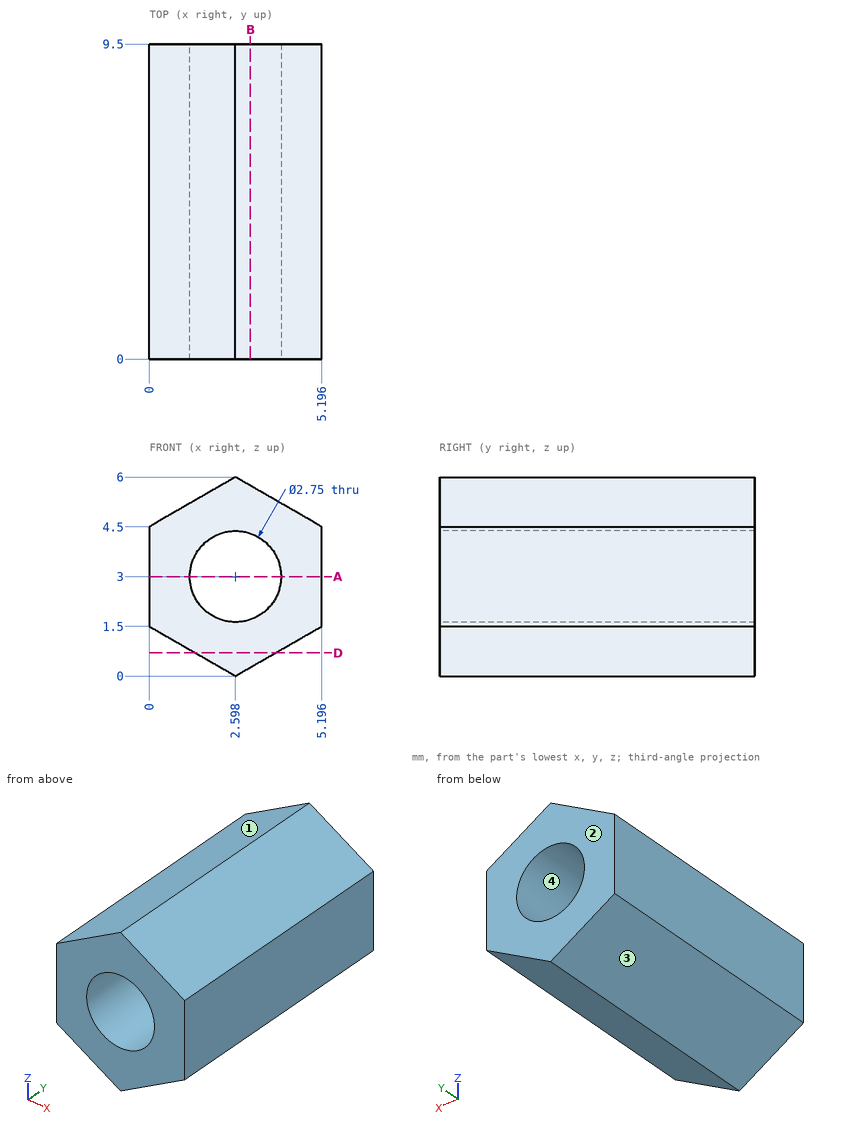
Input: dimensioned drawing with shaded views. Units: mm. Origin: part minimum x, y, z. Round coordinates to 2 decimals unless told otherwise and drop trailing zeros. Order: outer loops, then holes, each group sorted by start corner. A loop starts at its lowest first (then second) coordinate and runs counter-clockwise, first axis right, second up. Notation, with made-up numbers: (2.25, -25.5) -> (29.25, -25.5) arc R34 cw to (29.25, 6.5) -> close; hole circle Ø6 at (63.25, 86). An arc over 180 degrees is marked (long way). Put each result on its own line as item: value. Start each with the question number.
Q1. First-contact query: pin 1 (3 mm diameter, centred on x = 4.5, y = 1.5, fed in from +Z); pin 2 (2 mm diameter, centred on x = 1.5, y = 8, fed in from +Z). Flat tips, straight axial feed; report the tip coordinate or a pass-through.
Q2. Section A-A on z = 3. Return the cut outline in (x, y).
Q3. Section B-B on x = 3.05. Return the cut outline in (y, z).
Q4. Pull-direction query (Z, two-part tool) for the marked faces 1, 2, 3 and 4; classes: +Z half, -Z half, draft (parallel to the pull), parting line (faces both ways), or undercut.
Q5. Line query: probe 1 along Z at (x, y) = (2.2, 2.75); probe 2 along X at (y, z) = (7.5, 2) (1 decimal); probe 3 along Z at (x, y) = (3.4, 7). Output: solid intervals per line, ascending.
Q6. Section D-D on z = 0.7. Return the cut outline in (x, y).
Ans:
1. pin 1: stops at z = 5.77
1. pin 2: stops at z = 5.94
2. outline: (0, 0) -> (1.22, 0) -> (1.22, 9.5) -> (0, 9.5) -> close; (3.97, 0) -> (5.2, 0) -> (5.2, 9.5) -> (3.97, 9.5) -> close
3. outline: (0, 0.26) -> (9.5, 0.26) -> (9.5, 1.7) -> (0, 1.7) -> close; (0, 4.3) -> (9.5, 4.3) -> (9.5, 5.74) -> (0, 5.74) -> close
4. face 1: +Z half
4. face 2: draft
4. face 3: -Z half
4. face 4: undercut
5. probe 1: z = 0.23 to 1.68, 4.32 to 5.77
5. probe 2: x = 0 to 1.7, 3.5 to 5.2
5. probe 3: z = 0.46 to 1.88, 4.12 to 5.54
6. outline: (1.39, 0) -> (3.81, 0) -> (3.81, 9.5) -> (1.39, 9.5) -> close
